Read the model definition and answer for the solid it produces. Units are mm, in the model's axes. Face numbers are marked on the shaded views. A direction names the side the tool comes from. Round coordinates to 2 decimals unless told otherwise and drop trailing zeros. Order: outer loops, then holes, each group sorted by start corner. A loop starts at its lowest first (then second) coordinate and runs counter-clockwise, first axis right, second up. Notation, with made-up numbers: (8.5, 89.5) - (33.5, 89.5) arc R32 cw to (33.5, 119.5) - close; hole circle Ø3 at (-5.5, 13.5). An arc over 180 degrees is marked (long way). Put each result on its own line as item: value. Start each with the question number.
Q1. Section C-C on y = 2.5 is taken. Give the vertices of the cut face in (x, z), then the cut area to 3 significant figures.
Q2. Each of these flat-tipped pins is pushed along its axis until it touches: pin 1 Ø1.5 at (x, z) = (1.5, -2.5) entering from -Y; pin 2 Ø0.8 at (y, z) = (9.5, -2.5) entering from -X; pin 3 Ø0.7 at (x, z) = (0, 0.5) entering from +Y. Where does it stop, or does it pass through?
Q3. Section A-A on x = 0 is taken. Give the vertices of the cut face in (y, z).
Q4. Which of the six approach directions +Z, -Z, +X, -X, +Y, -Y give full straight-line access (tool end or side, diameter ignored) to the marked faces 1, 2, 3, 4 and 5?
Q5. Find the intervals of material crossed by line 1 along Z through (x, y) = (0, 8); line 2 along Y through (x, z) = (-1.4, 2.25), in increasing order. Write a range as from..to.
Q6. Section B-B on z = 0 is taken. Give the vertices of the cut face in (x, y), then the cut area to 3 significant figures.
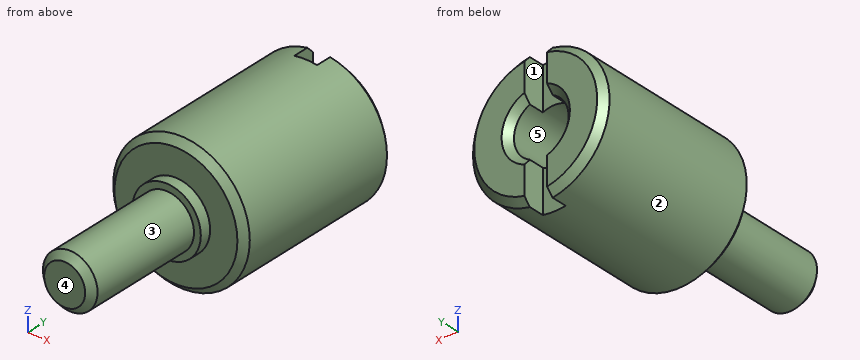
Autodesk Inventor part; units mm, degrees
ref_plane "YZ Plane" through (0, 0, 0) normal (1, 0, 0) x (0, 1, 0)
ref_plane "XZ Plane" through (0, 0, 0) normal (0, 1, 0) x (-1, 0, 0)
ref_plane "XY Plane" through (0, 0, 0) normal (0, 0, 1) x (1, 0, 0)
sketch "スケッチ1" plane through (0, 0, 0) normal (0, 0, 1) x (1, 0, 0)
  line L0 (0, -4) -> (0.9, -4)
  line L1 (0.9, -4) -> (1.2, -3.7)
  line L2 (1.2, -3.7) -> (1.2, 1.5)
  line L3 (1.2, 1.5) -> (1.5, 1.5)
  line L4 (1.5, 1.5) -> (1.5, 2)
  line L5 (1.5, 2) -> (2.7, 2)
  line L6 (3, 9.7) -> (2.7, 10)
  line L7 (2.7, 10) -> (1.5, 10)
  line L8 (1.5, 10) -> (1.2, 9.7)
  line L9 (0, 7.4044) -> (0, -7.4044) construction
  line L10 (0, -4) -> (0, 4)
  line L11 (0, 4) -> (1.2, 4)
  line L12 (1.2, 4) -> (1.2, 9.7)
  line L13 (2.7, 2) -> (3, 2.3)
  line L14 (3, 2.3) -> (3, 9.7)
  point P0 (0, 0)
  point P1 (0, 0)
  point P2 (0, 0)
  dimension "d0" = 2.4
  dimension "d1" = 6
  dimension "d2" = 0.3
  dimension "d3" = 0.3
  dimension "d4" = 3
  dimension "d5" = 0.5
  dimension "d6" = 8
  dimension "d7" = 0.3
  dimension "d8" = 2.4
  dimension "d9" = 6
  dimension "d10" = 0.3
  dimension "d11" = 0.3
  dimension "d12" = 0.3
  dimension "d13" = 0.3
  dimension "d14" = 6
revolve "回転1" add sketch "スケッチ1" angle 360 about axis through (0, 7.4044, 0) along (0, -1, 0)
sketch "スケッチ2" plane through (0, 10, 0) normal (0, 1, 0) x (1, 0, 0)
  line L0 (-0.5, 3) -> (0.5, 3)
  line L1 (0.5, 3) -> (0.5, -3)
  line L2 (0.5, -3) -> (-0.5, -3)
  line L3 (-0.5, -3) -> (-0.5, 3)
  line L4 (-0.5, 3) -> (0.5, -3) construction
  line L5 (0.5, 3) -> (-0.5, -3) construction
  circle A0 centre (0, 0) radius 3
  point P0 (0, 0)
  point P1 (0.5, 2.958)
  point P2 (-0.5, 2.958)
  point P3 (-0.5, -2.958)
  point P4 (0.5, -2.958)
  dimension "d16" = 1
extrude "押し出し1" cut sketch "スケッチ2" against normal blind 1 contours A0 L1 L3
equation "\"d3\" = d2"
equation "\"d10\" = d7"
equation "\"d11\" = d7"
equation "\"d12\" = d11"
equation "\"d13\" = d12"
properties part number "BRU-307S" material "ステンレス鋼 AISI 304"
Findings:
1. outline: circle Ø6 at (0, 0)
1. area: 28.3 mm2
2. pin 1: y = 2
2. pin 2: x = -2.14
2. pin 3: y = 4
3. outline: (-4, -0.9) - (-3.7, -1.2) - (1.5, -1.2) - (1.5, -1.5) - (2, -1.5) - (2, -2.7) - (2.3, -3) - (9, -3) - (9, -1.2) - (4, -1.2) - (4, 1.2) - (9, 1.2) - (9, 3) - (2.3, 3) - (2, 2.7) - (2, 1.5) - (1.5, 1.5) - (1.5, 1.2) - (-3.7, 1.2) - (-4, 0.9) - close
4. face 1: +Z, -Z, +Y
4. face 2: +Y, -Y
4. face 3: -Y
4. face 4: +Z, -Z, +X, -X, -Y
4. face 5: +Y
5. line 1: -3..-1.2, 1.2..3
5. line 2: 2..10
6. outline: (-3, 2.3) - (-2.7, 2) - (-1.5, 2) - (-1.5, 1.5) - (-1.2, 1.5) - (-1.2, -3.7) - (-0.9, -4) - (0.9, -4) - (1.2, -3.7) - (1.2, 1.5) - (1.5, 1.5) - (1.5, 2) - (2.7, 2) - (3, 2.3) - (3, 9.7) - (2.7, 10) - (1.5, 10) - (1.2, 9.7) - (1.2, 4) - (-1.2, 4) - (-1.2, 9.7) - (-1.5, 10) - (-2.7, 10) - (-3, 9.7) - close
6. area: 47.9 mm2
